Could you check a few things on this model? Use its own coordinates, in mm. Face numbers are marked on the shaded views. A direction names the side the tool comes from. Give positions to 0.01 mm unless a question says otherwise; leave off trailing zeros. Write each loop counter-clockwise with the first axis right and the second up, starting at its lowest first coordinate (ties: lowest second). Pieces come first, ordered by that corner, then holes. Notation, with made-up numbers: M 88.5,28.25 L 117.5,28.25 A20 cw 117.5,61.25 Z; hole C 40,75.25 d4. An arc over 180 degrees is marked long. One line per item, written item: value.
```python
from build123d import *

# Parameters (mm, degrees)
F0_W     = 28
F0_H     = 80
F1_DEPTH = 1
F0_W_2   = 1
F2_DEPTH = 15
F4_DEPTH = 28


with BuildPart() as f1:
    # F0 (on Top) → F1 (new body)
    with BuildSketch(Plane.XY):
        Rectangle(F0_W, F0_H)
    extrude(amount=F1_DEPTH)

    # F0 (on Top) → F2 (join)
    with BuildSketch(Plane.XY):
        with Locations((-14.5, 0)):
            Rectangle(F0_W_2, F0_H)
        with Locations((14.5, 0)):
            Rectangle(F0_W_2, F0_H)
    extrude(amount=F2_DEPTH)

    # F3 (on face) → F4 (join, through all)
    with BuildSketch(Plane.YZ.offset(-14)):
        Polygon((19.005928, 1), (20.005928, 1), (40, 15), (39, 15), align=None)
        Polygon((-0.300263, 1), (0.699737, 1), (20.693809, 15), (19.693809, 15), align=None)
        Polygon((-19.606455, 1), (-18.606455, 1), (1.387617, 15), (0.387617, 15), align=None)
        Polygon((-38.912646, 1), (-37.912646, 1), (-17.918574, 15), (-18.918574, 15), align=None)
    extrude(amount=F4_DEPTH)


solid = f1.part
```
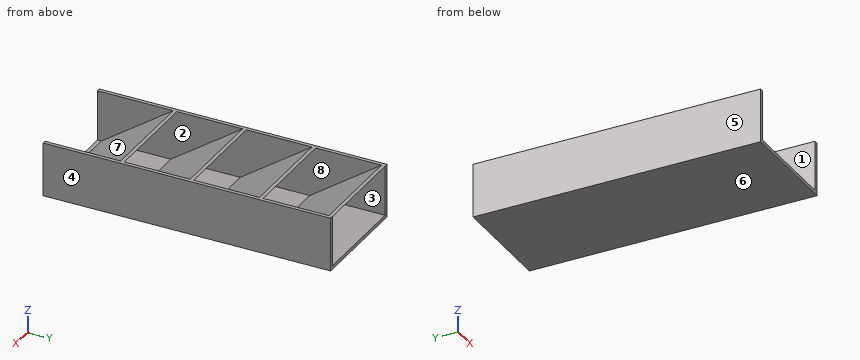
1) If we section it at A-A, the plane x = 3.5: Write out the boundary of the cut face in (y, z).
Outcome:
outline: M -40,0 L 40,0 L 40,1 L 20.01,1 L 40,15 L 39,15 L 19.01,1 L 0.7,1 L 20.69,15 L 19.69,15 L -0.3,1 L -18.61,1 L 1.39,15 L 0.39,15 L -19.61,1 L -37.91,1 L -17.92,15 L -18.92,15 L -38.91,1 L -40,1 Z
2) If we section it at B-B, the plane y = -27: Write out the boundary of the cut face in (x, z), then the cut area to 3 significant figures.
Outcome:
outline: M -15,0 L 15,0 L 15,15 L 14,15 L 14,9.34 L -14,9.34 L -14,15 L -15,15 Z; hole M -14,1 L 14,1 L 14,8.64 L -14,8.64 Z
area: 77.6 mm^2
3) Please list where these lines run through material, in increasing order: L1, parallel to X at y = -31.5, z = 8.25; L2, parallel to Y at x = 13.5, z = 4; L3, parallel to Y at x = -6.25, z = 3.25. Write a range as from..to.
Outcome:
L1: x = -15..-14, 14..15
L2: y = -34.63..-33.63, -15.32..-14.32, 3.98..4.98, 23.29..24.29
L3: y = -35.7..-34.7, -16.39..-15.39, 2.91..3.91, 22.22..23.22
4) If we section it at C-C, the plane z = 9.75: Write out the boundary of the cut face in (x, y).
Outcome:
outline: M -15,-40 L -14,-40 L -14,-26.42 L 14,-26.42 L 14,-40 L 15,-40 L 15,40 L 14,40 L 14,32.5 L -14,32.5 L -14,40 L -15,40 Z; hole M -14,-25.42 L 14,-25.42 L 14,-7.11 L -14,-7.11 Z; hole M -14,-6.11 L 14,-6.11 L 14,12.2 L -14,12.2 Z; hole M -14,13.2 L 14,13.2 L 14,31.5 L -14,31.5 Z
5) On a 3-axis mill with a long thin cutter (end or side, diameter ignored), from which of +Z, -Z, +X, -X, +Y, -Y can I reach the whole of each face in a straight line? I mean the marked faces 1, 2, 3 and 4. Say none if no direction works.
Outcome:
face 1: +Z, -Y
face 2: none
face 3: +Y
face 4: +Z, -Z, +X, +Y, -Y
6) We'd pull the mould along X, two halves only. Please class the marked faces 5, 6, 7 and 8: pulls with the +X half, pulls with the -X half, needs draft (parallel to the pull), parting line crosses it, or undercut.
Outcome:
face 5: pulls with the -X half
face 6: needs draft
face 7: undercut
face 8: undercut
7) I'm going to push flat-ended pins straight in: pin 1 (8 mm diameter, centred on x = 4, y = 14.5, fed in from +Z); pin 2 (12 mm diameter, centred on x = -6, y = -19, fed in from +Z); pin 3 (6 mm diameter, centred on x = -2, y = 27, fed in from +Z); pin 4 (6 mm diameter, centred on x = 6, z = 4.5, fed in from +Y). Where does each tip first touch, or does it pass through?
Outcome:
pin 1: stops at z = 14.16
pin 2: stops at z = 15
pin 3: stops at z = 8.7
pin 4: stops at y = 29.29
